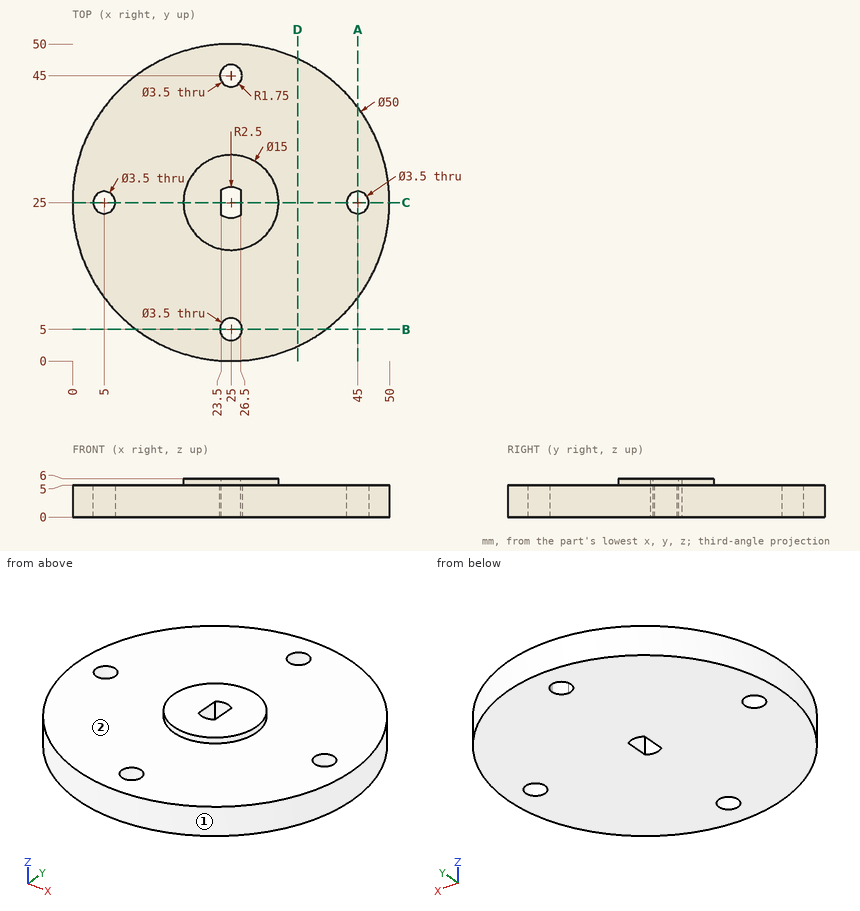
Verification items for this drawing (mm, ordinates from the low corner). Give positions to 0.01 mm unless a question says otherwise; leave off trailing zeros. Loops run counter-clockwise (first coordinate to the right, second up) from the corner with the lowest first, then second, coordinate; pieces in that order, holes last. Notation, with made-up numbers: M 87.5,-14.5 L 134.5,-14.5 A29 ccw 134.5,14.5 Z; hole C 17,-3.5 d5. An arc over 180 degrees is marked long. Answer as a JSON object with one key per item and string values. Group by question number.
Item 1: Gauge pin test, flat ends, axial feed: pin 1 (2 mm diameter, centred on y = 17.5, z = 4, fed in from -X); pin 2 (10 mm diameter, centred on x = 43.5, y = 37.5, fed in from +Z). Record the tip position at first contact, or that the pin passes through.
Item 2: Sectioned sample at C-C on y = 25. Record the boundary of the cut face in (x, z), plus the area to 3 significant figures.
Item 3: Material ranges on L1, parallel to Y at x = 25, z = 3.95; L2, parallel to Z at x = 13, y = 24; L3, parallel to Y at x = 25.5, z = 4.05 (3 decimals), recorded low to high.
Item 4: Sectioned sample at A-A on x = 45. Record the boundary of the cut face in (y, z).
Item 5: Sectioned sample at D-D on x = 35.5. Record the boundary of the cut face in (y, z), plus the area to 3 significant figures.
Item 6: Mould release check, pull along Y, two halves, no side actions. Record for the marked faces 1 and 2: pulls with the +Y half, pulls with the -Y half, needs draft (parallel to the pull), parting line crosses it, or undercut.
Findings below:
{
 "1": {"pin 1": "x = 0.86", "pin 2": "z = 5"},
 "2": {"outline": "M 0,0 L 3.25,0 L 3.25,5 L 0,5 Z; M 6.75,0 L 23.5,0 L 23.5,6 L 17.5,6 L 17.5,5 L 6.75,5 Z; M 26.5,0 L 43.25,0 L 43.25,5 L 32.5,5 L 32.5,6 L 26.5,6 Z; M 46.75,0 L 50,0 L 50,5 L 46.75,5 Z", "area": "212 mm2"},
 "3": {"L1": "0 to 3.25, 6.75 to 22.5, 27.5 to 43.25, 46.75 to 50", "L2": "0 to 5", "L3": "0.005 to 3.323, 6.677 to 22.551, 27.449 to 43.323, 46.677 to 49.995"},
 "4": {"outline": "M 10,0 L 23.25,0 L 23.25,5 L 10,5 Z; M 26.75,0 L 40,0 L 40,5 L 26.75,5 Z"},
 "5": {"outline": "M 2.31,0 L 47.69,0 L 47.69,5 L 2.31,5 Z", "area": "227 mm2"},
 "6": {"face 1": "parting line crosses it", "face 2": "needs draft"}
}
